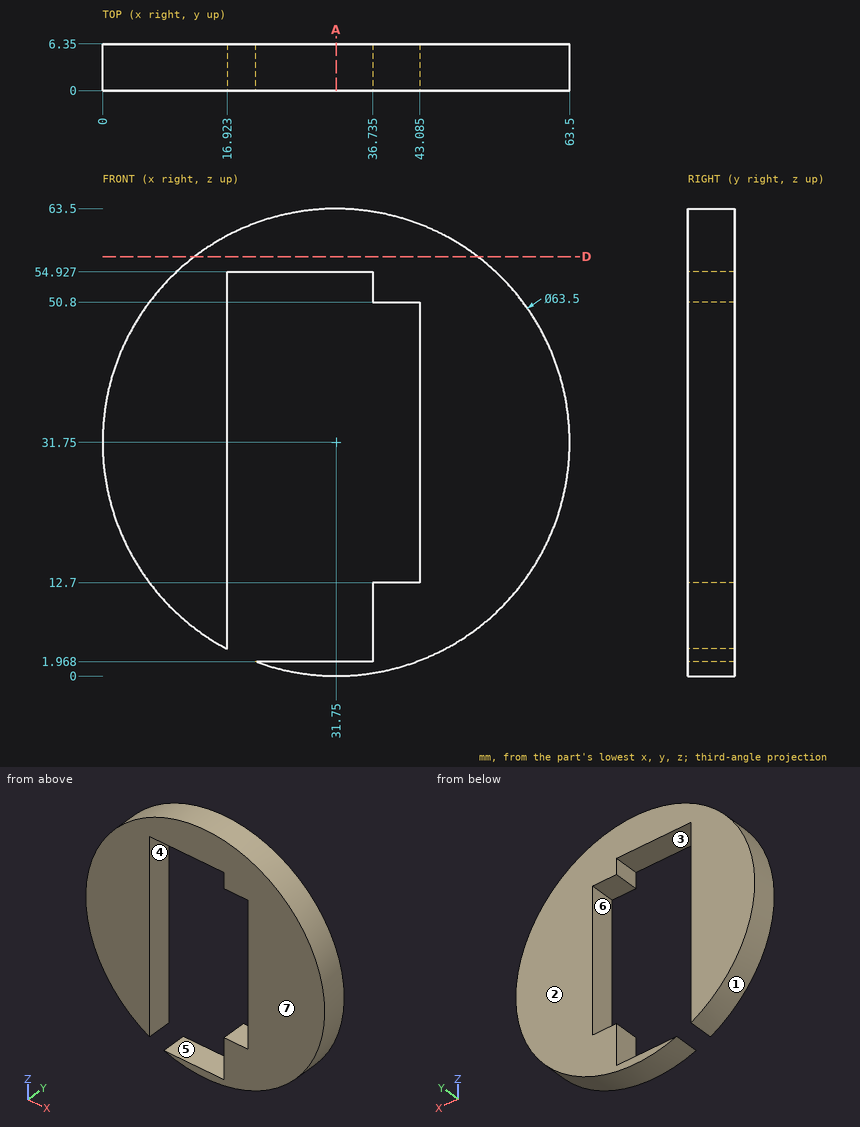
Could you check a few things on this drawing? It's one solid part, dimensions in mm from its lowest x, y, z. A direction names the side the tool comes from. Round coordinates to 2 decimals unless told otherwise and drop trailing zeros. Order: outer loops, then holes, each group sorted by start corner. A loop starts at its lowest first (then second) coordinate and runs counter-clockwise, first axis right, second up. Notation, with made-up numbers: M 80.5,6.25 L 139.5,6.25 A23 cw 139.5,36.25 Z; hole C 29.5,32.5 d11. An arc over 180 degrees is marked long. One line per item, written item: value.
(1) Imagine slicing it at A-A (x = 31.75). Write out the boundary of the cut face in (y, z).
Ans:
outline: M 0,0 L 6.35,0 L 6.35,1.97 L 0,1.97 Z; M 0,54.93 L 6.35,54.93 L 6.35,63.5 L 0,63.5 Z
(2) Which directions (+Z, -Z, +X, -X, +Y, -Y) give clear straight access to the entire face, cutting with the end or side of a thin tool? Please do the marked faces 4, 5, 6 and 7.
Ans:
face 4: -Z, +Y, -Y
face 5: -X, +Y, -Y
face 6: +Y, -Y
face 7: +Z, -Z, +X, -X, -Y
(3) If we mould it in two halves opening along Z, with no side actions, what happens to the marked faces 1, 2 and 3? For each: released by +Z, released by -Z, zero draft, split by the parting line, or undercut.
Ans:
face 1: split by the parting line
face 2: zero draft
face 3: undercut
(4) Imagine slicing it at D-D (z = 57). Write out the boundary of the cut face in (x, y).
Ans:
outline: M 12.5,0 L 51,0 L 51,6.35 L 12.5,6.35 Z
(5) I need wall thicknesses on line 1 along X through (y, z) = (5, 13) (1 decimal); line 2 along X through (y, z) = (3.75, 19.5) (1 decimal); line 3 along Z through (x, y) = (28, 5). Which ranges of each line are inside material? Lowest first, please. Write a range as from..to.
Ans:
line 1: x = 6.1..16.9, 43.1..57.4
line 2: x = 2.5..16.9, 43.1..61
line 3: z = 0.22..1.97, 54.93..63.28
(6) I'm going to push flat-ended pins straight in: P1, Ø1.5, axis at y = 2.5, z = 57, coming from the -X side (1 decimal); P2, Ø2, axis at x = 42.5, y = 1, coming from the +Z side (1 decimal); P3, Ø1.5, axis at y = 1, z = 22.5, coming from the -X side. Where does each tip first touch, or does it pass through?
Ans:
P1: stops at x = 11.6
P2: stops at z = 62
P3: stops at x = 1.16
